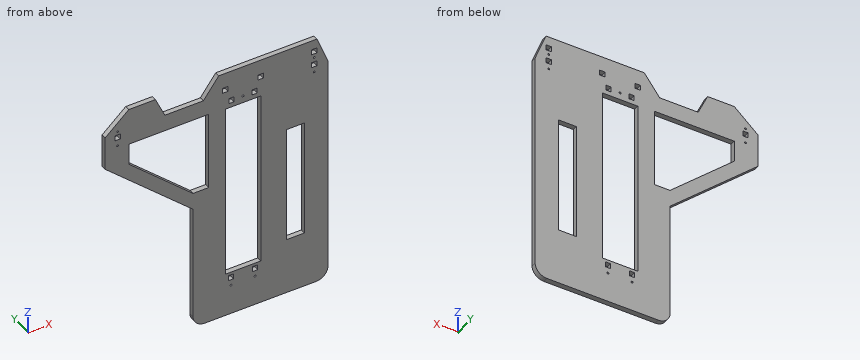
from build123d import *

# Parameters (mm, degrees)
BOSS_EXTRUDE1_DEPTH = 8.4
SKETCH2_R           = 1.5
SKETCH2_R_2         = 1.75
SKETCH2_W           = 60
SKETCH2_H           = 300
SKETCH2_W_2         = 9
SKETCH2_H_2         = 9
CUT_EXTRUDE1_DEPTH  = 9.4
FILLET1_R           = 20
SKETCH4_W           = 30
SKETCH4_H           = 200
CUT_EXTRUDE3_DEPTH  = 9.4


with BuildPart() as part:
    # Sketch1 → Boss-Extrude1 (new body)
    with BuildSketch(Plane(origin=(0, 0, 0), x_dir=(1, 0, 0), z_dir=(0, 1, 0))):
        Polygon((0, 0), (-228, 0), (-228, -215), (-376.5, -347.47169509), (-376.5, -404.47169509), (-336.5, -439.9), (-291.5, -439.9), (-275.5, -405), (-210.5, -405), (-184.5, -439.9), (-18.5, -439.9), (0, -392.4), align=None)
    extrude(amount=BOSS_EXTRUDE1_DEPTH)

    # Sketch2 → Cut-Extrude1 (cut, through all)
    with BuildSketch(Plane(origin=(0, 8.4, 0), x_dir=(1, 0, 0), z_dir=(0, 1, 0))):
        with Locations((-23.1, -408.2)):
            Circle(SKETCH2_R)
        with Locations((-23.1, -382)):
            Circle(SKETCH2_R)
        with Locations((-355.4, -407.37169509)):
            Circle(SKETCH2_R)
        with Locations((-355.4, -381.77169509)):
            Circle(SKETCH2_R)
        with Locations((-163.85, -51.1)):
            Circle(SKETCH2_R_2)
        with Locations((-123.15, -51.1)):
            Circle(SKETCH2_R_2)
        with Locations((-143.5, -387)):
            Circle(SKETCH2_R_2)
        Polygon((-336.5, -340.600531429), (-228, -243.811447811), (-201.5, -243.811447811), (-201.5, -377), (-336.5, -377), align=None)
        with Locations((-143.5, -224.9)):
            Rectangle(SKETCH2_W, SKETCH2_H)
        with Locations((-23.1, -419.4)):
            Rectangle(SKETCH2_W_2, SKETCH2_H_2)
        with Locations((-23.1, -395.95)):
            Rectangle(SKETCH2_W_2, SKETCH2_H_2)
        with Locations((-355.4, -396.97169509)):
            Rectangle(SKETCH2_W_2, SKETCH2_H_2)
        with Locations((-163.85, -65.6)):
            Rectangle(SKETCH2_W_2, SKETCH2_H_2)
        with Locations((-123.15, -65.6)):
            Rectangle(SKETCH2_W_2, SKETCH2_H_2)
        with Locations((-163, -387)):
            Rectangle(SKETCH2_W_2, SKETCH2_H_2)
        with Locations((-124, -387)):
            Rectangle(SKETCH2_W_2, SKETCH2_H_2)
        with Locations((-173.4, -410)):
            Rectangle(SKETCH2_W_2, SKETCH2_H_2)
        with Locations((-113.6, -410)):
            Rectangle(SKETCH2_W_2, SKETCH2_H_2)
    extrude(amount=-CUT_EXTRUDE1_DEPTH, mode=Mode.SUBTRACT)

    # Fillet1
    fillet1_edges = [part.edges().sort_by_distance(p)[0] for p in [
        (-228, 4.2, 0),
        (0, 4.2, 0),
    ]]
    fillet(fillet1_edges, radius=FILLET1_R)

    # Sketch4 → Cut-Extrude3 (cut, through all)
    with BuildSketch(Plane(origin=(0, 8.4, 0), x_dir=(1, 0, 0), z_dir=(0, 1, 0))):
        with Locations((-54.735091888, -195.993725651)):
            Rectangle(SKETCH4_W, SKETCH4_H)
    extrude(amount=-CUT_EXTRUDE3_DEPTH, mode=Mode.SUBTRACT)


solid = part.part
Work out the finished part from the listing and answer in its coordinate system (mm). Round coordinates to 2 decimals unless told otherwise and drop trailing zeros. Loops run counter-clockwise (first coordinate to the right, second up) from the corner with the lowest first, then second, coordinate; pieces in that order, holes last. Notation, with made-up numbers: (58, 84.5) -> (105, 84.5) arc R37 cw to (105, 120.5) -> close; hole circle Ø7 at (66.5, -35.75). An arc over 180 degrees is marked (long way). Use one line per item in the form item = value.
(1) Straight lines are drawn through the part: line 1 (Z direction, x = -23.1, y = 2.75); line 2 (Z direction, x = -163.85, y = 6); line 3 (X direction, y = 6, z = 51.1). For each, find the intervals that lie inside material, in ascending order.
Answer list:
line_1 = 0 to 380.5, 383.5 to 391.45, 400.45 to 406.7, 409.7 to 414.9, 423.9 to 439.9
line_2 = 0 to 49.35, 52.85 to 61.1, 70.1 to 74.9, 374.9 to 382.5, 391.5 to 439.9
line_3 = -228 to -165.6, -162.1 to -124.9, -121.4 to 0
(2) Flat-ended cylindrical pins translate along their axes: P1, Ø3, axis at x = -260, y = 3.5, coming from the +Z side; P2, Ø4, axis at x = -354.5, y = 2.5, coming from the +Z side. Find the tip coordinate at first contact, or state that the pin passes through.
Answer list:
P1 = 405
P2 = 425.73
(3) Find section D-D on y = 4. Give the number of separate pieces and of enclosed holes in the cut face, then the cut area to 3 significant figures.
Answer list:
separate_pieces = 1
enclosed_holes = 19
area = 82,000 mm2
(4) Find section B-B on x = -281. Give the vertices of the cut face in (y, z).
Answer list:
outline = (0, 262.28) -> (8.4, 262.28) -> (8.4, 291.09) -> (0, 291.09) -> close; (0, 377) -> (8.4, 377) -> (8.4, 417) -> (0, 417) -> close
(5) Find section A-A on z = 199.5. Give the vertices of the cut face in (x, y).
Answer list:
outline = (-228, 0) -> (-173.5, 0) -> (-173.5, 8.4) -> (-228, 8.4) -> close; (-113.5, 0) -> (-69.74, 0) -> (-69.74, 8.4) -> (-113.5, 8.4) -> close; (-39.74, 0) -> (0, 0) -> (0, 8.4) -> (-39.74, 8.4) -> close
(6) Find section C-C on z = 328. Give the vertices of the cut face in (x, y), then the cut area to 3 significant figures.
Answer list:
outline = (-354.67, 0) -> (-322.37, 0) -> (-322.37, 8.4) -> (-354.67, 8.4) -> close; (-201.5, 0) -> (-173.5, 0) -> (-173.5, 8.4) -> (-201.5, 8.4) -> close; (-113.5, 0) -> (0, 0) -> (0, 8.4) -> (-113.5, 8.4) -> close
area = 1,460 mm2
